CAD build for the part. Positions are in the model's coordinates, mm. A direction names the side the tool comes from. Round coordinates to 2 decimals unless told otherwise and drop trailing zeros. Loops run counter-clockwise (first coordinate to the right, second up) from the corner with the lowest first, then second, coordinate; pieces in that order, holes last. Notation, with made-up numbers: M 81.5,-24 L 136.5,-24 A35 ccw 136.5,8 Z; hole C -15.75,-25 d9. An arc over 180 degrees is marked long. One line per item, written item: value. Start each with the question number.
from build123d import *

# Parameters (mm, degrees)
SKETCH2_W                      = 150
SKETCH2_H                      = 150
BOSS_EXTRUDE1_DEPTH            = 30
SKETCH3_W                      = 80
SKETCH3_H                      = 80
BOSS_EXTRUDE2_DEPTH            = 40
SKETCH4_W                      = 150
SKETCH4_H                      = 150
BOSS_EXTRUDE3_DEPTH            = 20
HOLE1_D                        = 26
HOLE1_DEPTH                    = 100
HOLE1_CBORE_D                  = 60
HOLE1_CBORE_DEPTH              = 10
M16_TAPPED_HOLE2_D             = 14
M16_TAPPED_HOLE2_DEPTH         = 30
F_10_0_10_DIAMETER_HOLE1_D     = 10
F_10_0_10_DIAMETER_HOLE1_DEPTH = 16
F_10_0_10_DIAMETER_HOLE1_TIP   = 3.004303095
CHAMFER1_SIZE                  = 2


with BuildPart() as part:
    # Sketch2 → Boss-Extrude1 (new body)
    with BuildSketch(Plane(origin=(0, 0, 0), x_dir=(1, 0, 0), z_dir=(0, 1, 0))):
        Rectangle(SKETCH2_W, SKETCH2_H)
    extrude(amount=-BOSS_EXTRUDE1_DEPTH)

    # Sketch3 → Boss-Extrude2 (add)
    with BuildSketch(Plane.XZ.offset(30)):
        Rectangle(SKETCH3_W, SKETCH3_H)
    extrude(amount=BOSS_EXTRUDE2_DEPTH)

    # Sketch4 → Boss-Extrude3 (add)
    with BuildSketch(Plane.XZ.offset(70)):
        Rectangle(SKETCH4_W, SKETCH4_H)
    extrude(amount=BOSS_EXTRUDE3_DEPTH)

    # Hole1
    with Locations(Plane(origin=(0, -90, 0), x_dir=(-1, 0, 0), z_dir=(0, -1, 0))):
        with Locations((0, 0)):
            CounterBoreHole(HOLE1_D / 2, HOLE1_CBORE_D / 2, HOLE1_CBORE_DEPTH, depth=HOLE1_DEPTH)

    # M16 Tapped Hole2
    with Locations(Plane(origin=(0, 0, 0), x_dir=(1, 0, 0), z_dir=(0, 1, 0))):
        with Locations((60, -60), (-60, 60), (-60, -60), (60, 60), (0, 60), (-60, 0), (0, -60), (60, 0)):
            Hole(M16_TAPPED_HOLE2_D / 2, depth=M16_TAPPED_HOLE2_DEPTH)

    # Ø10.0 (10) Diameter Hole1
    with Locations(Plane(origin=(0, -90, 0), x_dir=(-1, 0, 0), z_dir=(0, -1, 0))):
        with Locations((-52, 0), (0, -52), (52, 0), (0, 52)):
            Hole(F_10_0_10_DIAMETER_HOLE1_D / 2, depth=F_10_0_10_DIAMETER_HOLE1_DEPTH)
            with Locations((0, 0, -(F_10_0_10_DIAMETER_HOLE1_DEPTH + F_10_0_10_DIAMETER_HOLE1_TIP / 2))):  # 118° drill point
                Cone(0, F_10_0_10_DIAMETER_HOLE1_D / 2, F_10_0_10_DIAMETER_HOLE1_TIP, mode=Mode.SUBTRACT)

    # Chamfer1
    chamfer1_edges = [part.edges().sort_by_distance(p)[0] for p in [
        (30, -90, 0),
    ]]
    chamfer(chamfer1_edges, length=CHAMFER1_SIZE)


solid = part.part
(1) Slice it at D-D, the plane x = -60. List the corners of the cut face in (y, z).
(2) Slice it at A-A, the plane z = 60. List the corners of the cut face in (x, y).
(3) Flat gauge pins, fed straight in: P1, Ø22.5, axis at x = -60, z = 60, coming from the +Y side; P2, Ø9, axis at x = 52, z = 0, coming from the -Y side; P3, Ø10, axis at y = -35.5, z = 46, coming from the -X side; P4, Ø12, axis at x = 8.5, z = -16.5, coming from the -Y side. Where does each tip first touch, or does it go through?
(4) Slice it at B-B, the plane y = -17. Count the separate pieces of the cut face and the enclosed holes in it, and give its area (3 significant figures).
(5) Mould opens along Z. For faces 1 (the conical face through (52.69, -71.52, 0.53)), 2 (the flat face through (-1, -50, 40)), 3 (the flat face through (-1, -15, -75)) say: pulls with the +Z half, pulls with the -Z half, needs draft (parallel to the pull), parting line crosses it, or undercut.
(6) Probe L1, parallel to X at y = -17, z = -60; L2, parallel to Z at x = 0, y = -78.5. List the from-to ranges inside material, lowest first.
(7) Which spindle directions (+Z, -Z, +X, -X, +Y, -Y) get a long thin tool onto all of the face, cutting with end or side? Do faces 4 (the cylindrical face through (-59.09, -15.21, -66.94)), 5 (the cylindrical face through (29.97, -84.06, -1.32)), 6 (the flat face through (-1, -50, -40)). Say none if no direction does.
(8) Slice it at C-C, the plane x = 34. List the corners of the cut face in (y, z).
Check result:
1. outline: M -90,-75 L -70,-75 L -70,75 L -90,75 Z; M -30,-75 L 0,-75 L 0,-67 L -30,-67 Z; M -30,-53 L 0,-53 L 0,-7 L -30,-7 Z; M -30,7 L 0,7 L 0,53 L -30,53 Z; M -30,67 L 0,67 L 0,75 L -30,75 Z
2. outline: M -75,-90 L 75,-90 L 75,-70 L -75,-70 Z; M -75,-30 L -67,-30 L -67,0 L -75,0 Z; M -53,-30 L -7,-30 L -7,0 L -53,0 Z; M 7,-30 L 53,-30 L 53,0 L 7,0 Z; M 67,-30 L 75,-30 L 75,0 L 67,0 Z
3. P1: stops at y = 0
3. P2: stops at y = -73.7
3. P3: passes through
3. P4: stops at y = -80
4. separate pieces: 1
4. enclosed holes: 9
4. area: 20,700 mm^2
5. face 1: undercut
5. face 2: pulls with the +Z half
5. face 3: pulls with the -Z half
6. L1: x = -75 to -67, -53 to -7, 7 to 53, 67 to 75
6. L2: z = -75 to -57, -47 to -13, 13 to 47, 57 to 75
7. face 4: +Y
7. face 5: -Y
7. face 6: -Z, +X, -X
8. outline: M -90,-75 L -70,-75 L -70,-40 L -30,-40 L -30,-75 L 0,-75 L 0,75 L -30,75 L -30,40 L -70,40 L -70,75 L -90,75 Z
